from build123d import *

# Parameters (mm, degrees)
SKETCH1_R           = 8
SKETCH1_R_2         = 7
BOSS_EXTRUDE1_DEPTH = 467.66
SCALE1_SCALE        = 0.857142857


with BuildPart() as part:
    # Sketch1 → Boss-Extrude1 (new body)
    with BuildSketch(Plane(origin=(0, 0, 0), x_dir=(1, 0, 0), z_dir=(0, 1, 0))):
        with Locations(Location((0, 0, 0), (0, 0, 270))):
            Circle(SKETCH1_R)
        with Locations(Location((0, 0, 0), (0, 0, 270))):
            Circle(SKETCH1_R_2, mode=Mode.SUBTRACT)
    extrude(amount=BOSS_EXTRUDE1_DEPTH)

    # Sketch2 → Revolve1 (revolve)
    with BuildSketch(Plane.XY, mode=Mode.PRIVATE) as revolve1_sk:
        with BuildLine():
            Line((8, 2), (8.5, 2))
            ThreePointArc((8.5, 2), (9.5, 3), (8.5, 4))
            Line((8.5, 4), (8, 4))
            Line((8, 4), (8, 2))
        make_face()
    revolve(revolve1_sk.sketch.rotate(Axis((0, 0, 0), (0, 1, 0)), 90), axis=Axis((0, 0, 0), (0, 1, 0)))


with BuildPart() as part_1:
    # Scale1: scaled about (0, 232.373730032, 0)
    add(part.part.scale(SCALE1_SCALE).moved(Location((0, 33.196247147, 0))))


solid = part_1.part
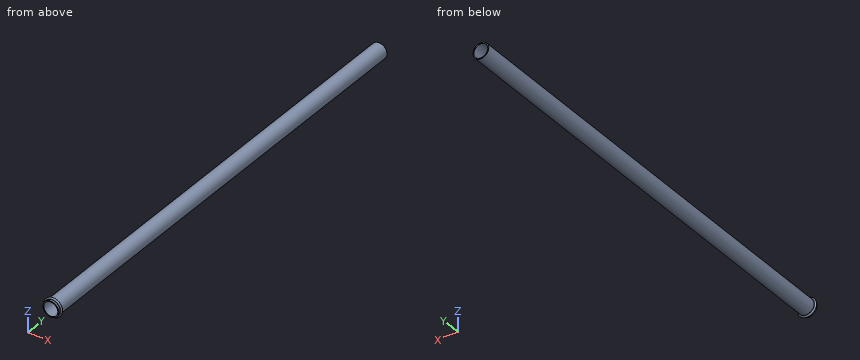
Build history of the part. All positions in model axes, mm. Coordinates: 2 decimals unless noted, no trailing zeros. Write each loop counter-clockwise with the first axis right and the second up, starting at its lowest first coordinate (ties: lowest second). Pieces come first, ordered by that corner, then holes.
(1) Cut at A-A on z = 0. List the corners of the cut face in (x, y), and give its area (3 significant figures).
(2) Cut at C-C on y = 68. List the corners of the cut face in (x, z), and give its area (3 significant figures).
(3) Drill centre lines: line 1 (X direction, y = 209, z = 0); line 2 (Z direction, x = 3.25, y = 278); line 3 (Z direction, x = 5.5, y = 293). Where is each one in solid material? Low to high.
(4) Pin check, flat tips, straight feed: pin 1 Ø5 at (x, y) = (5.5, 338.5) entering from -Z; pin 2 Ø2 at (y, z) = (392, -5.5) entering from +X; pin 3 Ø2 at (y, z) = (183, 4) entering from +X. Stop position of each tip, or through.
(5) Cut at B-B on x = 0. List the corners of the cut face in (y, z).
Working result:
1. outline: (-7.29, 34.91) - (-6.86, 34.91) - (-6.86, 33.2) - (-6, 33.2) - (-6, 434.05) - (-6.86, 434.05) - (-6.86, 36.62) - (-7.29, 36.62) arc R0.86 ccw to start; (6, 33.2) - (6.86, 33.2) - (6.86, 34.91) - (7.29, 34.91) arc R0.86 ccw to (7.29, 36.62) - (6.86, 36.62) - (6.86, 434.05) - (6, 434.05) - close
1. area: 691 mm2
2. outline: circle Ø13.71 at (0, 0); hole circle Ø12 at (0, 0)
2. area: 34.6 mm2
3. line 1: x = -6.86 to -6, 6 to 6.86
3. line 2: z = -6.04 to -5.04, 5.04 to 6.04
3. line 3: z = -4.1 to -2.4, 2.4 to 4.1
4. pin 1: stops at z = -6.17
4. pin 2: stops at x = 5.17
4. pin 3: stops at x = 6.17
5. outline: (33.2, -6.86) - (34.91, -6.86) - (34.91, -7.29) arc R0.86 ccw to (36.62, -7.29) - (36.62, -6.86) - (434.05, -6.86) - (434.05, -6) - (33.2, -6) - close; (33.2, 6) - (434.05, 6) - (434.05, 6.86) - (36.62, 6.86) - (36.62, 7.29) arc R0.86 ccw to (34.91, 7.29) - (34.91, 6.86) - (33.2, 6.86) - close
